Here's how the part is built. I have some questions about the finished solid (model axes, mm). Round coordinates to 2 decimals unless told otherwise and drop trailing zeros. Loops run counter-clockwise (first coordinate to the right, second up) from the corner with the lowest first, then second, coordinate; pieces in that order, holes last. Notation, with made-up numbers: (27.5, 79) - (81.5, 79) arc R23 cw to (81.5, 92) - close; hole circle Ø11 at (36.25, 32). An arc over 180 degrees is marked (long way). Return JSON: item names as keys, results as strings. Group by question number.
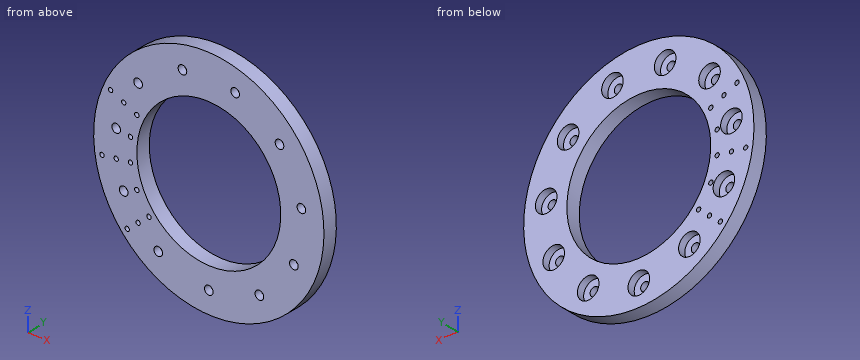
```python
from build123d import *

# Parameters (mm, degrees)
SKETCH1_R               = 80
BOSS_EXTRUDE1_DEPTH     = 10
SKETCH3_R               = 3
CUT_EXTRUDE1_DEPTH      = 10
SKETCH4_R               = 7.5
CUT_EXTRUDE2_DEPTH      = 5
SKETCH5_R               = 50
CUT_EXTRUDE3_DEPTH      = 21
CUT_EXTRUDE4_DEPTH      = 114.578166916
CUT_EXTRUDE4_DEPTH_BACK = 114.578166916
SKETCH6_R               = 1.5


with BuildPart() as part:
    # Sketch1 → Boss-Extrude1 (new body)
    with BuildSketch(Plane(origin=(0, 0, 0), x_dir=(1, 0, 0), z_dir=(0, 1, 0))):
        with Locations(Location((0, 0, 0), (0, 0, 270))):
            Circle(SKETCH1_R)
    extrude(amount=BOSS_EXTRUDE1_DEPTH)

    # Sketch3 → Cut-Extrude1 (cut)
    with BuildSketch(Plane(origin=(0, 10, 0), x_dir=(1, 0, 0), z_dir=(0, 1, 0))):
        with Locations(Location((0, 65, 0), (0, 0, 270))):
            Circle(SKETCH3_R)
        with Locations(Location((35.141653135, 54.681479634, 0), (0, 0, 270))):
            Circle(SKETCH3_R)
        with Locations(Location((59.126079698, 27.001975845, 0), (0, 0, 270))):
            Circle(SKETCH3_R)
        with Locations(Location((64.338393722, -9.250464488, 0), (0, 0, 270))):
            Circle(SKETCH3_R)
        with Locations(Location((49.123722333, -42.565947706, 0), (0, 0, 270))):
            Circle(SKETCH3_R)
        with Locations(Location((18.312616195, -62.367043285, 0), (0, 0, 270))):
            Circle(SKETCH3_R)
        with Locations(Location((-18.312616195, -62.367043285, 0), (0, 0, 270))):
            Circle(SKETCH3_R)
        with Locations(Location((-49.123722333, -42.565947706, 0), (0, 0, 270))):
            Circle(SKETCH3_R)
        with Locations(Location((-64.338393722, -9.250464488, 0), (0, 0, 270))):
            Circle(SKETCH3_R)
        with Locations(Location((-59.126079698, 27.001975845, 0), (0, 0, 270))):
            Circle(SKETCH3_R)
        with Locations(Location((-35.141653135, 54.681479634, 0), (0, 0, 270))):
            Circle(SKETCH3_R)
    extrude(amount=-CUT_EXTRUDE1_DEPTH, mode=Mode.SUBTRACT)

    # Sketch4 → Cut-Extrude2 (cut)
    with BuildSketch(Plane(origin=(0, 10, 0), x_dir=(1, 0, 0), z_dir=(0, 1, 0))):
        with Locations(Location((0, 65, 0), (0, 0, 270))):
            Circle(SKETCH4_R)
        with Locations(Location((35.141653135, 54.681479634, 0), (0, 0, 270))):
            Circle(SKETCH4_R)
        with Locations(Location((59.126079698, 27.001975845, 0), (0, 0, 270))):
            Circle(SKETCH4_R)
        with Locations(Location((64.338393722, -9.250464488, 0), (0, 0, 270))):
            Circle(SKETCH4_R)
        with Locations(Location((49.123722333, -42.565947706, 0), (0, 0, 270))):
            Circle(SKETCH4_R)
        with Locations(Location((18.312616195, -62.367043285, 0), (0, 0, 270))):
            Circle(SKETCH4_R)
        with Locations(Location((-18.312616195, -62.367043285, 0), (0, 0, 270))):
            Circle(SKETCH4_R)
        with Locations(Location((-49.123722333, -42.565947706, 0), (0, 0, 270))):
            Circle(SKETCH4_R)
        with Locations(Location((-64.338393722, -9.250464488, 0), (0, 0, 270))):
            Circle(SKETCH4_R)
        with Locations(Location((-59.126079698, 27.001975845, 0), (0, 0, 270))):
            Circle(SKETCH4_R)
        with Locations(Location((-35.141653135, 54.681479634, 0), (0, 0, 270))):
            Circle(SKETCH4_R)
    extrude(amount=-CUT_EXTRUDE2_DEPTH, mode=Mode.SUBTRACT)

    # Sketch5 → Cut-Extrude3 (cut)
    with BuildSketch(Plane(origin=(0, 10, 0), x_dir=(1, 0, 0), z_dir=(0, 1, 0))):
        with Locations(Location((0, 0, 0), (0, 0, 270))):
            Circle(SKETCH5_R)
    extrude(amount=-CUT_EXTRUDE3_DEPTH, mode=Mode.SUBTRACT)

    # Sketch6 → Cut-Extrude4 (cut, two sides: drawn at the far end of the back side and taken through both)
    with BuildSketch(Plane(origin=(0, 10, 0), x_dir=(1, 0, 0), z_dir=(0, 1, 0)).offset(-CUT_EXTRUDE4_DEPTH_BACK)):
        with Locations(Location((-56.681218077, 49.114555046, 0), (0, 0, 270))):
            Circle(SKETCH6_R)
        with Locations(Location((-49.123722333, 42.565947706, 0), (0, 0, 270))):
            Circle(SKETCH6_R)
        with Locations(Location((-41.566226589, 36.017340367, 0), (0, 0, 270))):
            Circle(SKETCH6_R)
        with Locations(Location((-54.43918532, 7.834226299, 0), (0, 0, 270))):
            Circle(SKETCH6_R)
        with Locations(Location((-64.337219014, 9.258631081, 0), (0, 0, 270))):
            Circle(SKETCH6_R)
        with Locations(Location((-74.235252709, 10.683035863, 0), (0, 0, 270))):
            Circle(SKETCH6_R)
        with Locations(Location((-50.03555842, -22.83512412, 0), (0, 0, 270))):
            Circle(SKETCH6_R)
        with Locations(Location((-59.132932678, -26.986964869, 0), (0, 0, 270))):
            Circle(SKETCH6_R)
        with Locations(Location((-68.230306936, -31.138805619, 0), (0, 0, 270))):
            Circle(SKETCH6_R)
        with Locations(Location((-50.029759744, 22.847825715, 0), (0, 0, 270))):
            Circle(SKETCH6_R)
        with Locations(Location((-54.440179303, -7.827316105, 0), (0, 0, 270))):
            Circle(SKETCH6_R)
    extrude(amount=CUT_EXTRUDE4_DEPTH + CUT_EXTRUDE4_DEPTH_BACK, mode=Mode.SUBTRACT)


solid = part.part
```
Q1. Imagine slicing it at B-B, the plane z = -65. List the corners of the cut face in (x, y) for me.
Q2. Imagine slicing it at D-D, the plane z = 52. List the corners of the cut face in (x, y) for me.
Q3. Imagine slicing it at C-C, the plane y = 3.5. Give the number of separate pieces and of enclosed holes in the cut face, and give its area (3 significant figures).
Q4. Imagine slicing it at A-A, the plane x = 0. List the corners of the cut face in (y, z) for me.
Q5. Will these pins go through, and if not, where does the flat tip stop? pin 1 Ø2 at (x, y) = (49, 7.5) entering from +Z; pin 2 Ø12 at (x, z) = (59.13, -27) entering from +Y; pin 3 Ø6 at (x, y) = (-22.5, 6.5) entering from +Z.
Q6. Please list where these lines run through material, in increasing order: line 1 (X direction, y = 8.5, z = 4.5); line 2 (X direction, y = 7.25, z = 65.5); line 3 (Z direction, x = -23, y = 9).
Output values:
{
 "1": {"outline": "(-46.64, 0) - (-3, 0) - (-3, 5) - (-7.5, 5) - (-7.5, 10) - (-46.64, 10) - close; (3, 0) - (46.64, 0) - (46.64, 10) - (7.5, 10) - (7.5, 5) - (3, 5) - close"},
 "2": {"outline": "(-60.79, 0) - (60.79, 0) - (60.79, 10) - (-60.79, 10) - close"},
 "3": {"separate pieces": "1", "enclosed holes": "23", "area": "11,900 mm^2"},
 "4": {"outline": "(0, -80) - (10, -80) - (10, -72.5) - (5, -72.5) - (5, -68) - (0, -68) - close; (0, -62) - (5, -62) - (5, -57.5) - (10, -57.5) - (10, -50) - (0, -50) - close; (0, 50) - (10, 50) - (10, 80) - (0, 80) - close"},
 "5": {"pin 1": "stops at z = 64", "pin 2": "stops at y = 5", "pin 3": "stops at z = 77.59"},
 "6": {"line 1": "x = -79.87 to -70.14, -58.53 to -49.8, 49.8 to 58.53, 70.14 to 79.87", "line 2": "x = -45.93 to -25.13, -11.5 to 11.5, 25.13 to 45.93", "line 3": "z = -76.62 to -44.4, 44.4 to 56.51, 68.22 to 76.62"}
}
